The model under review builds one solid part; all positions refer to its coordinate system, in mm. A direction names the side the tool comes from. Round coordinates to 2 decimals unless told otherwise and drop trailing zeros. Write each loop counter-clockwise with the first axis right and the second up, starting at its lowest first coordinate (ties: lowest second). Pieces come first, ordered by that corner, then holes. Notation, with made-up numbers: (86, 89) - (97, 89) arc R15 ccw to (97, 103) - close; hole circle Ø8 at (-31, 46.5). An arc over 180 degrees is marked (long way). Write each question's results on one line, items separated by ' | '.
```python
from build123d import *

# Parameters (mm, degrees)
SKETCH1_R                  = 1.5
BASE_FLANGE2_DEPTH         = 3
CUT_EXTRUDE1_DEPTH         = 3
FILLET2_R                  = 3
SKETCHED_START             = -72.08
SKETCHED_BEND2_OUTLINE_W   = 139.27076518
SKETCHED_BEND2_OUTLINE_H   = 3
SKETCHED_BEND2_DEPTH       = 11.04
SKETCHED_START_2           = -11.04
SKETCHED_BEND2_2_OUTLINE_W = 139.27076518
SKETCHED_BEND2_2_OUTLINE_H = 3
SKETCHED_BEND2_2_DEPTH     = 11.04
SKETCHED_START_3           = -60.687339692
SKETCHED_BEND2_3_OUTLINE_W = 139.27076518
SKETCHED_BEND2_3_OUTLINE_H = 11.999956935
SKETCHED_BEND2_3_OUTLINE_R = 1.5
SKETCHED_BEND2_3_DEPTH     = 2.647339692
SKETCHED_START_4           = -14.04
SKETCHED_BEND2_4_OUTLINE_W = 139.27076518
SKETCHED_BEND2_4_OUTLINE_H = 11.999956935
SKETCHED_BEND2_4_OUTLINE_R = 1.5
SKETCHED_BEND2_4_DEPTH     = 2.616101716
SKETCHED_START_5           = -14.7766
SKETCHED_BEND2_5_OUTLINE_W = 139.27076518
SKETCHED_BEND2_5_OUTLINE_H = 11.999956935
SKETCHED_BEND2_5_OUTLINE_R = 1.5
SKETCHED_BEND2_5_DEPTH     = 3.7366
SKETCHED_START_6           = -61.04
SKETCHED_BEND2_6_OUTLINE_W = 139.27076518
SKETCHED_BEND2_6_OUTLINE_H = 11.999956935
SKETCHED_BEND2_6_OUTLINE_R = 1.5
SKETCHED_BEND2_6_DEPTH     = 3.7366
SKETCHED_START_7           = -140
SKETCHED_BEND2_7_DEPTH     = 141


with BuildPart() as part:
    # Base-Flange2: sheet metal written as solids
    # Sketch1 → Base-Flange2 (new body)
    with BuildSketch(Plane.XY):
        Polygon((-72.08, -139.27076518), (-28.43, -139.27076518), (-22.43, -139.27076518), (0, -139.27076518), (0, 0), (-22.43, 0), (-28.43, 0), (-72.08, 0), align=None)
        with Locations((-25.43, -134.27076518)):
            Circle(SKETCH1_R, mode=Mode.SUBTRACT)
        with Locations((-25.43, -76.20135678)):
            Circle(SKETCH1_R, mode=Mode.SUBTRACT)
        with Locations((-25.43, -63.0694084)):
            Circle(SKETCH1_R, mode=Mode.SUBTRACT)
        with Locations((-25.43, -5)):
            Circle(SKETCH1_R, mode=Mode.SUBTRACT)
        with Locations((-64.58, -69.63538259)):
            Circle(SKETCH1_R, mode=Mode.SUBTRACT)
        with Locations((-64.58, -105.23606098)):
            Circle(SKETCH1_R, mode=Mode.SUBTRACT)
        with Locations((-64.58, -34.0347042)):
            Circle(SKETCH1_R, mode=Mode.SUBTRACT)
        with Locations(Location((-7.5, -105.23606098, 0), (0, 0, 180))):
            Circle(SKETCH1_R, mode=Mode.SUBTRACT)
        with Locations(Location((-7.5, -69.63538259, 0), (0, 0, 180))):
            Circle(SKETCH1_R, mode=Mode.SUBTRACT)
        with Locations(Location((-7.5, -34.0347042, 0), (0, 0, 180))):
            Circle(SKETCH1_R, mode=Mode.SUBTRACT)
    extrude(amount=-BASE_FLANGE2_DEPTH)

    # Sketch16 → Cut-Extrude1 (cut)
    with BuildSketch(Plane.XY):
        Polygon((-56.04, -3), (-56.04, -14.774529578), (-44.735, -63.055915667), (-31.43, -6.232930978), (-31.43, -3), align=None)
        Polygon((-31.43, -19.391864824), (-43.194429615, -69.63538259), (-31.43, -119.878900356), align=None)
        Polygon((-46.275570385, -69.63538259), (-56.04, -27.933463424), (-56.04, -111.337301756), align=None)
        Polygon((-44.735, -76.214849513), (-56.04, -124.496235602), (-56.04, -136.27076518), (-31.43, -136.27076518), (-31.43, -133.037834202), align=None)
    extrude(amount=-CUT_EXTRUDE1_DEPTH, mode=Mode.SUBTRACT)

    # Fillet2
    fillet2_edges = [part.edges().sort_by_distance(p)[0] for p in [
        (-31.43, -136.27076518, -1.5),
        (-44.735, -76.214849513, -1.5),
        (-56.04, -124.496235602, -1.5),
        (-56.04, -136.27076518, -1.5),
        (-56.04, -3, -1.5),
        (-56.04, -14.774529578, -1.5),
        (-44.735, -63.055915667, -1.5),
        (-31.43, -3, -1.5),
        (-31.43, -19.391864824, -1.5),
        (-43.194429615, -69.63538259, -1.5),
        (-31.43, -119.878900356, -1.5),
        (-56.04, -111.337301756, -1.5),
        (-46.275570385, -69.63538259, -1.5),
        (-56.04, -27.933463424, -1.5),
    ]]
    fillet(fillet2_edges, radius=FILLET2_R)

    # Sketched Bend2: read off the stored shape, not the designer's step
    # Sketched Bend2 outline → Sketched Bend2 (cut)
    with BuildSketch(Plane.YZ.offset(SKETCHED_START)):
        with Locations((-69.63538259, -1.5)):
            Rectangle(SKETCHED_BEND2_OUTLINE_W, SKETCHED_BEND2_OUTLINE_H)
    extrude(amount=SKETCHED_BEND2_DEPTH, mode=Mode.SUBTRACT)

    # Sketched Bend2 2 outline → Sketched Bend2 2 (cut)
    with BuildSketch(Plane.YZ.offset(SKETCHED_START_2)):
        with Locations((-69.63538259, -1.5)):
            Rectangle(SKETCHED_BEND2_2_OUTLINE_W, SKETCHED_BEND2_2_OUTLINE_H)
    extrude(amount=SKETCHED_BEND2_2_DEPTH, mode=Mode.SUBTRACT)

    # Sketched Bend2 3 outline → Sketched Bend2 3 (add)
    with BuildSketch(Plane.YZ.offset(SKETCHED_START_3)):
        with Locations((-69.63538259, 5.999978468)):
            Rectangle(SKETCHED_BEND2_3_OUTLINE_W, SKETCHED_BEND2_3_OUTLINE_H)
        with Locations((-105.23606098, 4.499956935)):
            Circle(SKETCHED_BEND2_3_OUTLINE_R, mode=Mode.SUBTRACT)
        with Locations((-69.63538259, 4.499956935)):
            Circle(SKETCHED_BEND2_3_OUTLINE_R, mode=Mode.SUBTRACT)
        with Locations((-34.0347042, 4.499956935)):
            Circle(SKETCHED_BEND2_3_OUTLINE_R, mode=Mode.SUBTRACT)
    extrude(amount=SKETCHED_BEND2_3_DEPTH)

    # Sketched Bend2 4 outline → Sketched Bend2 4 (add)
    with BuildSketch(Plane.YZ.offset(SKETCHED_START_4)):
        with Locations((-69.63538259, 5.999978468)):
            Rectangle(SKETCHED_BEND2_4_OUTLINE_W, SKETCHED_BEND2_4_OUTLINE_H)
        with Locations((-105.23606098, 4.499956935)):
            Circle(SKETCHED_BEND2_4_OUTLINE_R, mode=Mode.SUBTRACT)
        with Locations((-69.63538259, 4.499956935)):
            Circle(SKETCHED_BEND2_4_OUTLINE_R, mode=Mode.SUBTRACT)
        with Locations((-34.0347042, 4.499956935)):
            Circle(SKETCHED_BEND2_4_OUTLINE_R, mode=Mode.SUBTRACT)
    extrude(amount=SKETCHED_BEND2_4_DEPTH)

    # Sketched Bend2 5 outline → Sketched Bend2 5 (add)
    with BuildSketch(Plane.YZ.offset(SKETCHED_START_5)):
        with Locations((-69.63538259, 5.999978468)):
            Rectangle(SKETCHED_BEND2_5_OUTLINE_W, SKETCHED_BEND2_5_OUTLINE_H)
        with Locations((-105.23606098, 4.499956935)):
            Circle(SKETCHED_BEND2_5_OUTLINE_R, mode=Mode.SUBTRACT)
        with Locations((-69.63538259, 4.499956935)):
            Circle(SKETCHED_BEND2_5_OUTLINE_R, mode=Mode.SUBTRACT)
        with Locations((-34.0347042, 4.499956935)):
            Circle(SKETCHED_BEND2_5_OUTLINE_R, mode=Mode.SUBTRACT)
    extrude(amount=SKETCHED_BEND2_5_DEPTH)

    # Sketched Bend2 6 outline → Sketched Bend2 6 (add)
    with BuildSketch(Plane.YZ.offset(SKETCHED_START_6)):
        with Locations((-69.63538259, 5.999978468)):
            Rectangle(SKETCHED_BEND2_6_OUTLINE_W, SKETCHED_BEND2_6_OUTLINE_H)
        with Locations((-105.23606098, 4.499956935)):
            Circle(SKETCHED_BEND2_6_OUTLINE_R, mode=Mode.SUBTRACT)
        with Locations((-69.63538259, 4.499956935)):
            Circle(SKETCHED_BEND2_6_OUTLINE_R, mode=Mode.SUBTRACT)
        with Locations((-34.0347042, 4.499956935)):
            Circle(SKETCHED_BEND2_6_OUTLINE_R, mode=Mode.SUBTRACT)
    extrude(amount=SKETCHED_BEND2_6_DEPTH)

    # Sketched Bend2 7 outline → Sketched Bend2 7 (cut)
    with BuildSketch(Plane(origin=(0, 0, 0), x_dir=(1, 0, 0), z_dir=(0, 1, 0)).offset(SKETCHED_START_7)):
        with BuildLine():
            Line((-58.04, -0.7366), (-58.04, -11.999956935))
            Line((-58.04, -11.999956935), (-57.3034, -11.999956935))
            Line((-57.3034, -11.999956935), (-57.3034, 0))
            ThreePointArc((-57.3034, 0), (-57.824254855, -0.215745145), (-58.04, -0.7366))
        make_face()
        with BuildLine():
            Line((-14.7766, -11.999956935), (-14.04, -11.999956935))
            Line((-14.04, -11.999956935), (-14.04, -0.7366))
            ThreePointArc((-14.04, -0.7366), (-14.255745145, -0.215745145), (-14.7766, 0))
            Line((-14.7766, 0), (-14.7766, -11.999956935))
        make_face()
        with BuildLine():
            Line((-11.04, 3), (-14.7766, 3))
            ThreePointArc((-14.7766, 3), (-12.134424801, 1.905575199), (-11.04, -0.7366))
            Line((-11.04, -0.7366), (-11.04, 3))
        make_face()
        with BuildLine():
            ThreePointArc((-61.04, -0.7366), (-59.945575199, 1.905575199), (-57.3034, 3))
            Line((-57.3034, 3), (-61.04, 3))
            Line((-61.04, 3), (-61.04, -0.7366))
        make_face()
    extrude(amount=SKETCHED_BEND2_7_DEPTH, mode=Mode.SUBTRACT)


solid = part.part
```
Q1. We need section B-B (x = -25.43). State the section outline as (y, z) points, plus the area to 3 significant figures.
Evaluation:
outline: (-139.27, -3) - (-135.77, -3) - (-135.77, 0) - (-139.27, 0) - close; (-132.77, -3) - (-77.7, -3) - (-77.7, 0) - (-132.77, 0) - close; (-74.7, -3) - (-64.57, -3) - (-64.57, 0) - (-74.7, 0) - close; (-61.57, -3) - (-6.5, -3) - (-6.5, 0) - (-61.57, 0) - close; (-3.5, -3) - (0, -3) - (0, 0) - (-3.5, 0) - close | area: 382 mm^2
Q2. Tool access review of faces 1 (the flat face through (-61.04, -71, 6)), 2 (the flat face through (-44, -3, -1)): name each direction out of +Z, -Z, +X, -X, +Y, -Y from which nothing blocks a thin tool from reaching the whole face with its end or side.
Evaluation:
face 1: +Z, -Z, -X, +Y, -Y | face 2: +Z, -Z
Q3. We need section A-A (z = 9.75). State the section outline as (x, y) points, plus the area to 3 significant figures.
Evaluation:
outline: (-61.04, -139.27) - (-58.04, -139.27) - (-58.04, 0) - (-61.04, 0) - close; (-14.04, -139.27) - (-11.04, -139.27) - (-11.04, 0) - (-14.04, 0) - close | area: 836 mm^2
Q4. We need section C-C (y = -8.5). State the section outline as (x, z) points, plus the area to 3 significant figures.
Evaluation:
outline: (-61.04, 0.74) arc R3.74 ccw to (-57.3, -3) - (-56.04, -3) - (-56.04, 0) - (-57.3, 0) arc R0.74 cw to (-58.04, 0.74) - (-58.04, 12) - (-61.04, 12) - close; (-31.96, -3) - (-14.78, -3) arc R3.74 ccw to (-11.04, 0.74) - (-11.04, 12) - (-14.04, 12) - (-14.04, 0.74) arc R0.74 cw to (-14.78, 0) - (-31.96, 0) - close | area: 144 mm^2
Q5. The part is to be moulded in two halves that separate along Z. For faces 3 (the cylindrical face through (-44.791, -86.374, -1.521)), 4 (the cylindrical face through (-12.561, -32.604, 4.951)), 5 (the flat face through (-27, -69, 0)), say which applies: released by +Z, released by -Z, zero draft, split by the parting line, or undercut.
Evaluation:
face 3: zero draft | face 4: undercut | face 5: released by +Z
Q6. Insertion check: P1, Ø1.8, axis at x = -25.43, y = -134.27, coming from the +Z side; P2, Ø2.5, axis at y = -61.5, z = -1, coming from the -X side; P3, Ø10, axis at x = -46.5, y = -96, coming from the +Z side; P4, Ø0.9, axis at y = -129, z = -1.5, coming from the +X side. Each pin has a flat end and moves straight along its axis. Give the tip position at first contact, or say it passes through.
Evaluation:
P1: passes through | P2: stops at x = -61.01 | P3: stops at z = 0 | P4: stops at x = -11.49
Q7. For probe 1 along Y at (x, z) = (-25.43, -1.2); probe 2 along X at (y, z) = (-23, 5); probe 3 along Z at (x, y) = (-23, -14.5), list the stretches that pass through material, from the lowest coordinate up.
Evaluation:
probe 1: y = -139.27 to -135.77, -132.77 to -77.7, -74.7 to -64.57, -61.57 to -6.5, -3.5 to 0 | probe 2: x = -61.04 to -58.04, -14.04 to -11.04 | probe 3: z = -3 to 0
Q8. We need section D-D (x = -45). State the section outline as (y, z) points, plus the area to 3 significant figures.
Evaluation:
outline: (-139.27, -3) - (-136.27, -3) - (-136.27, 0) - (-139.27, 0) - close; (-86.39, -3) - (-52.89, -3) - (-52.89, 0) - (-86.39, 0) - close; (-3, -3) - (0, -3) - (0, 0) - (-3, 0) - close | area: 119 mm^2
